Check sheet for the modelled part. Datum: model origin and axes. Units: mm. A direction names the side the tool comes from. Coordinates: 2 decimals unless noted, no trailing zeros. Loops run counter-clockwise (first coordinate to the right, second up) from the corner with the lowest first, then second, coordinate; pieces in that order, holes last. Notation, with made-up numbers: (89.25, 73.25) - (99.25, 73.25) arc R24 cw to (99.25, 106.25) - close; hole circle Ø9 at (60.25, 17). An arc over 180 degrees is marked (long way). Write each question's results on one line, items separated by ' | '. Start each with the question number.
1. Cross-section at A-A (z = 9.25). Record the cut outline in (x, y), and give its area (3 significant figures).
2. Cross-section at D-D (x = -0.75). Record the cut outline in (y, z).
3. Tool access check on faces 1 (the face through (1.5, 2, -3)), 2 (the face through (-6, 2, 13)), 3 (the face through (2, 2, -0.2)). Record the directions out of +Z, -Z, +X, -X, +Y, -Y that give a thin tool (end or side, any length) a straight path to the whole face; none if there is none.
4. Gauge pin test, flat ends, axial feed: P1, Ø1, axis at x = 2, y = 2.5, coming from the -Z side; P2, Ø1.3, axis at x = 2, y = 1.5, coming from the +Z side; P3, Ø0.9, axis at x = -0.5, y = 2.5, coming from the +Z side. Record the tip position at first contact, or that the pin passes through.
5. Cross-section at C-C (z = -4.25). Record the cut outline in (x, y).
6. Thickness scan on line 1 (X direction, y = 0.8, z = 10); line 2 (X direction, y = 1.55, z = 2.75); line 3 (Z direction, x = -5.25, y = 2.95). Record the ranges inside material, lowest first. Write a range as [from, to].
Autodesk Inventor part; units mm, degrees
ref_plane "YZ Plane" through (0, 0, 0) normal (1, 0, 0) x (0, 1, 0)
ref_plane "XZ Plane" through (0, 0, 0) normal (0, 1, 0) x (-1, 0, 0)
ref_plane "XY Plane" through (0, 0, 0) normal (0, 0, 1) x (1, 0, 0)
sketch "Sketch1" plane through (0, 0, 0) normal (0, 1, 0) x (-1, 0, 0)
  line L0 (8, 13) -> (8, 7)
  line L1 (8, 7) -> (8, 7)
  line L2 (8, 7) -> (8, -13)
  line L3 (8, -13) -> (-8, -13)
  line L4 (-8, -13) -> (-8, 13)
  line L5 (-8, 13) -> (-4, 13)
  line L6 (-4, 13) -> (-4, 7)
  line L7 (-4, 7) -> (4, 7)
  line L8 (4, 7) -> (4, 13)
  line L9 (4, 13) -> (8, 13)
  line L10 (8, -13) -> (-8, 13) construction
  line L11 (1.5, 7) -> (-1.5, 7)
  line L12 (-1.5, 7) -> (-1.5, -5)
  line L13 (-1.5, -5) -> (1.5, -5)
  line L14 (1.5, -5) -> (1.5, 7)
  line L15 (2.7, -0.2) -> (-2.7, -0.2)
  line L16 (-2.7, -0.2) -> (-2.7, 2.2)
  line L17 (-2.7, 2.2) -> (2.7, 2.2)
  line L18 (2.7, 2.2) -> (2.7, -0.2)
  point P0 (0, 0)
  point P1 (0, 0)
  point P2 (0, 2.2)
  point P3 (0, -5)
  point P4 (-2.7, 1)
  point P5 (-1.5, 1)
  point P6 (0, 7)
  point P7 (1.5, 2.2)
  point P8 (1.5, -0.2)
  point P9 (-1.5, -0.2)
  point P10 (-1.5, 2.2)
  dimension "d0" = 6
  dimension "d1" = 4
  dimension "d3" = 0
  dimension "d4" = 4
  dimension "d5" = 20
  dimension "d10" = 8
  dimension "d11" = 3
  dimension "d12" = 12
  dimension "d13" = 5.4
  dimension "d14" = 2.4
extrude "Extrusion1" add sketch "Sketch1" along normal blind 4 contours L0 L2 L3 L4 L5 L6 L7 L12 L17 L16 L15 L13 L14 L18 L8 L9
fillet "Fillet1" radius 16 1 edges at (8, 2, -13)
properties part number "Lever" material "MDF Medium Density Fiberboard"
Established:
1) outline: (-8, 0) - (-4, 0) - (-4, 4) - (-8, 4) - close; (4, 0) - (8, 0) - (8, 4) - (4, 4) - close | area: 32.0 mm^2
2) outline: (0, -11.26) - (4, -11.26) - (4, -5) - (0, -5) - close
3) face 1: +Z, +Y, -Y | face 2: +Z, +X, -X, +Y, -Y | face 3: +Y, -Y
4) P1: z = -9.87 | P2: z = 7 | P3: z = -5
5) outline: (-8, 0) - (-1.5, 0) - (-1.5, 4) - (-8, 4) - close; (1.5, 0) - (6.26, 0) - (6.26, 4) - (1.5, 4) - close
6) line 1: [-8, -4], [4, 8] | line 2: [-8, -1.5], [1.5, 8] | line 3: [-12.76, 13]
